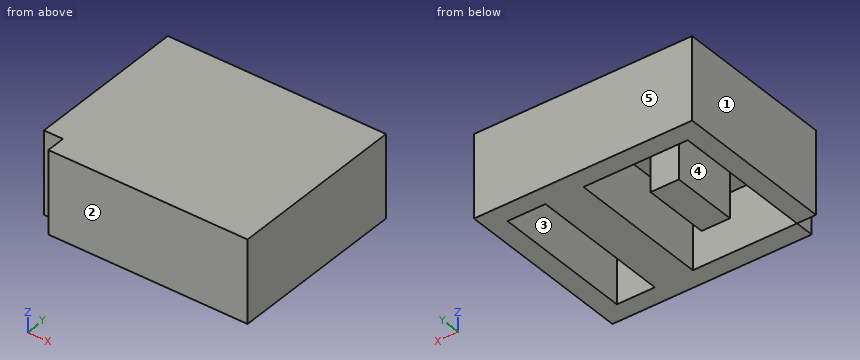
Autodesk Inventor part; units mm, degrees
ref_plane "YZ Plane" through (0, 0, 0) normal (1, 0, 0) x (0, 1, 0)
ref_plane "XZ Plane" through (0, 0, 0) normal (0, 1, 0) x (-1, 0, 0)
ref_plane "XY Plane" through (0, 0, 0) normal (0, 0, 1) x (1, 0, 0)
sketch "TopProfile" plane through (0, 0, 0) normal (0, 0, 1) x (1, 0, 0)
  line L0 (0, 19.6865) -> (0, 0)
  line L1 (9.1702, 14.4367) -> (5.2497, 14.4367)
  line L2 (5.2497, 14.4367) -> (5.2497, 5.2497)
  line L3 (5.2497, 5.2497) -> (9.1702, 5.2497)
  line L4 (9.1702, 5.2497) -> (9.1702, 14.4367)
  line L5 (19.6697, 0) -> (24.9194, 0)
  line L6 (24.9194, 0) -> (24.9194, 19.6865)
  line L7 (24.9194, 19.6865) -> (19.6697, 19.6865)
  line L8 (19.6697, 19.6865) -> (19.6697, 0)
  line L9 (-2.6249, 0) -> (-2.6249, 22.3113)
  line L10 (-2.6249, 22.3113) -> (27.5442, 22.3113)
  line L11 (27.5442, 22.3113) -> (27.5442, -2.6249)
  line L12 (27.5442, -2.6249) -> (0, -2.6249)
  line L13 (0, -2.6249) -> (0, 0)
  line L14 (0, 0) -> (-2.6249, 0)
  line L15 (14.4199, 0) -> (14.4199, 19.6865)
  line L16 (14.4199, 19.6865) -> (0, 19.6865)
  line L17 (0, 0) -> (14.4199, 0)
  line L18 (-2.6249, 0) -> (-2.6249, -2.6249)
  line L19 (-2.6249, -2.6249) -> (0, -2.6249)
  dimension "d3" = 3.9205
  dimension "d4" = 5.2497
  dimension "d8" = 5.2497
  dimension "d12" = 5.2497
  dimension "d13" = 2.6249
  dimension "d14" = 5.2497
  dimension "d15" = 5.2497
  dimension "d16" = 2.6249
  dimension "d17" = 2.6249
  dimension "d18" = 2.6249
  dimension "d19" = 24.9362
  dimension "d20" = 27.5443
  dimension "d21" = 5.2497
extrude "NegativeFeature" add sketch "TopProfile" against normal blind 11.43 contours L14 L9 L10 L11 L12 L13 | L4 L3 L2 L1
extrude "PositiveFeature" add sketch "TopProfile" against normal blind 3.175 contours L16 L15 L17 L0 | L8 L7 L6 L5
properties part number "switchback-logo-01"
For this review, take the finished solid that the model builds, in its own axes (mm). Face numbers are marked on the shaded views. A direction names the side the tool comes from. Give positions to 0.01 mm unless a question says otherwise; leave off trailing zeros. Order: outer loops, then holes, each group sorted by start corner. A loop starts at its lowest first (then second) coordinate and runs counter-clockwise, first axis right, second up.
1) Take a section at D-D (y = 0.5). Give the boundary of the cut face in (x, z) (3 decimals).
2) For the marked faces 4 and 5, list the 3-axis set-ups (+Z, -Z, +X, -X, +Y, -Y) from which the entire face can be reached by the end or side of a thin tool; tool diameter is ignored.
3) Insertion check: pin 1 (2.5 mm diameter, centred on x = 23, y = 11.5, fed in from -Z) (3 decimals); pin 2 (1.3 mm diameter, centred on y = -1.5, z = -8.5, fed in from -X). Each pin has a flat end and moves straight along its axis. Give the tip position at first contact, or say it passes through.
4) Wall thickness on line 1 (X direction, y = 14, z = -5.25); line 2 (X direction, y = 5, z = -5.75); line 3 (Y direction, x = 6, z = -9.5): over which ranges is each line inside the solid? List them lowest first.
5) The part is to be moulded in two halves that separate along X. For the marked faces 1, 2 and 3, say which applies: released by +X, released by -X, zero draft, split by the parting line, or undercut.
6) Take a section at B-B (y = 8). Give the boundary of the cut face in (x, z) (3 decimals), then the cut area to 3 significant figures.
7) Take a section at C-C (x = 22). Give the boundary of the cut face in (y, z) (1 decimal), then the cut area to 3 significant figures.
Derived:
1. outline: (-2.625, -11.43) - (0, -11.43) - (0, -3.175) - (14.42, -3.175) - (14.42, -11.43) - (19.67, -11.43) - (19.67, -3.175) - (24.919, -3.175) - (24.919, -11.43) - (27.544, -11.43) - (27.544, 0) - (-2.625, 0) - close
2. face 4: -Z
2. face 5: +Z, -Z, +X, -X, +Y
3. pin 1: stops at z = -3.175
3. pin 2: stops at x = 0
4. line 1: x = -2.62 to 0, 5.25 to 9.17, 14.42 to 19.67, 24.92 to 27.54
4. line 2: x = -2.62 to 0, 14.42 to 19.67, 24.92 to 27.54
4. line 3: y = -2.62 to 0, 5.25 to 14.44, 19.69 to 22.31
5. face 1: released by -X
5. face 2: zero draft
5. face 3: undercut
6. outline: (-2.625, -11.43) - (0, -11.43) - (0, -3.175) - (5.25, -3.175) - (5.25, -11.43) - (9.17, -11.43) - (9.17, -3.175) - (14.42, -3.175) - (14.42, -11.43) - (19.67, -11.43) - (19.67, -3.175) - (24.919, -3.175) - (24.919, -11.43) - (27.544, -11.43) - (27.544, 0) - (-2.625, 0) - close
6. area: 215 mm2
7. outline: (-2.6, -11.4) - (0, -11.4) - (0, -3.2) - (19.7, -3.2) - (19.7, -11.4) - (22.3, -11.4) - (22.3, 0) - (-2.6, 0) - close
7. area: 123 mm2
